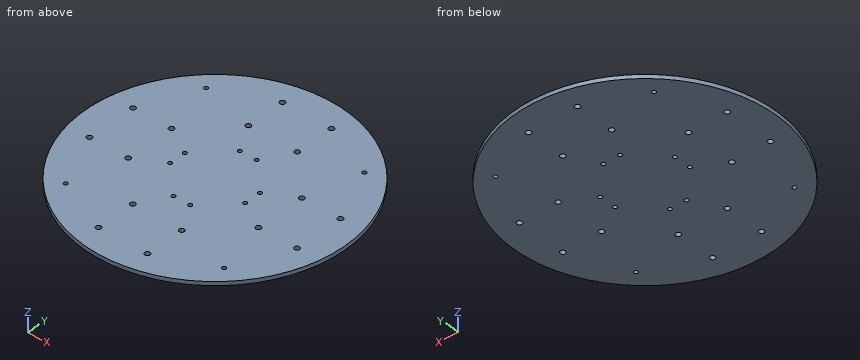
from build123d import *

# Parameters (mm, degrees)
CROQUIS1_R              = 100
CROQUIS1_R_2            = 2
SALIENTE_EXTRUIR1_DEPTH = 3
CORTAR_EXTRUIR2_START   = -3
CROQUIS2_R              = 2
CROQUIS2_R_2            = 1.5
CORTAR_EXTRUIR2_DEPTH   = 3
CROQUIS4_R              = 1.5
CORTAR_EXTRUIR3_DEPTH   = 3


with BuildPart() as part:
    # Croquis1 → Saliente-Extruir1 (new body)
    with BuildSketch(Plane.XY):
        Circle(CROQUIS1_R)
        with Locations((-50.610307618, 19)):
            Circle(CROQUIS1_R_2, mode=Mode.SUBTRACT)
        with Locations((-50.610307618, -19)):
            Circle(CROQUIS1_R_2, mode=Mode.SUBTRACT)
        with Locations((-80.610307618, 19)):
            Circle(CROQUIS1_R_2, mode=Mode.SUBTRACT)
        with Locations((-80.610307618, -19)):
            Circle(CROQUIS1_R_2, mode=Mode.SUBTRACT)
        with Locations((-19, -50.610307618)):
            Circle(CROQUIS1_R_2, mode=Mode.SUBTRACT)
        with Locations((19, -50.610307618)):
            Circle(CROQUIS1_R_2, mode=Mode.SUBTRACT)
        with Locations((-19, -80.610307618)):
            Circle(CROQUIS1_R_2, mode=Mode.SUBTRACT)
        with Locations((19, -80.610307618)):
            Circle(CROQUIS1_R_2, mode=Mode.SUBTRACT)
        with Locations((50.610307618, -19)):
            Circle(CROQUIS1_R_2, mode=Mode.SUBTRACT)
        with Locations((50.610307618, 19)):
            Circle(CROQUIS1_R_2, mode=Mode.SUBTRACT)
        with Locations((80.610307618, -19)):
            Circle(CROQUIS1_R_2, mode=Mode.SUBTRACT)
        with Locations((80.610307618, 19)):
            Circle(CROQUIS1_R_2, mode=Mode.SUBTRACT)
        with Locations((19, 50.610307618)):
            Circle(CROQUIS1_R_2, mode=Mode.SUBTRACT)
        with Locations((-19, 50.610307618)):
            Circle(CROQUIS1_R_2, mode=Mode.SUBTRACT)
        with Locations((19, 80.610307618)):
            Circle(CROQUIS1_R_2, mode=Mode.SUBTRACT)
        with Locations((-19, 80.610307618)):
            Circle(CROQUIS1_R_2, mode=Mode.SUBTRACT)
    extrude(amount=SALIENTE_EXTRUIR1_DEPTH)

    # Croquis2 → Cortar-Extruir2 (cut)
    with BuildSketch(Plane.XY.offset(3).offset(CORTAR_EXTRUIR2_START)):
        with Locations((19, 80.610307618)):
            Circle(CROQUIS2_R)
        with Locations((19, 50.610307618)):
            Circle(CROQUIS2_R)
        with Locations((-19, 50.610307618)):
            Circle(CROQUIS2_R)
        with Locations((-19, 80.610307618)):
            Circle(CROQUIS2_R)
        with Locations((-6.5, 29.110307618)):
            Circle(CROQUIS2_R_2)
        with Locations((6.5, 29.110307618)):
            Circle(CROQUIS2_R_2)
        with Locations((29.110307618, 6.5)):
            Circle(CROQUIS2_R_2)
        with Locations((29.110307618, -6.5)):
            Circle(CROQUIS2_R_2)
        with Locations((6.5, -29.110307618)):
            Circle(CROQUIS2_R_2)
        with Locations((-6.5, -29.110307618)):
            Circle(CROQUIS2_R_2)
        with Locations((-29.110307618, -6.5)):
            Circle(CROQUIS2_R_2)
        with Locations((-29.110307618, 6.5)):
            Circle(CROQUIS2_R_2)
    extrude(amount=CORTAR_EXTRUIR2_DEPTH, mode=Mode.SUBTRACT)

    # Croquis4 → Cortar-Extruir3 (cut)
    with BuildSketch(Plane.XY.offset(3)):
        with Locations((-61.518289963, 61.518289963)):
            Circle(CROQUIS4_R)
        with Locations((61.518289963, 61.518289963)):
            Circle(CROQUIS4_R)
        with Locations((61.518289963, -61.518289963)):
            Circle(CROQUIS4_R)
        with Locations((-61.518289963, -61.518289963)):
            Circle(CROQUIS4_R)
    extrude(amount=-CORTAR_EXTRUIR3_DEPTH, mode=Mode.SUBTRACT)


solid = part.part
Here's how the part is built. I have some questions about the finished solid (model axes, mm). Round coordinates to 2 decimals unless told otherwise and drop trailing zeros. Loops run counter-clockwise (first coordinate to the right, second up) from the corner with the lowest first, then second, coordinate; pieces in that order, holes last.
1. If we section it at A-A on z = 0.85: Count the separate pieces of the cut face and the enclosed holes in it, plus the area to 3 significant figures.
Answer list:
separate pieces: 1
enclosed holes: 28
area: 31,100 mm2
2. If I drill on line 1 along X through (y, z) = (82, 0.8); line 2 along Y through (x, z) = (6.5, 2.25); line 3 along Y through (x, z) = (-20, 2.5), over which ranges is the centre line in solid material (lowest first)?
Answer list:
line 1: x = -57.24 to -20.44, -17.56 to 17.56, 20.44 to 57.24
line 2: y = -99.79 to -30.61, -27.61 to 27.61, 30.61 to 99.79
line 3: y = -97.98 to -82.34, -78.88 to -52.34, -48.88 to 48.88, 52.34 to 78.88, 82.34 to 97.98
3. For P1, Ø2.5, axis at x = -19, y = -50.61, coming from the -Z side; P2, Ø1, axis at y = 16, z = 2, coming from the +X side, each with a flat end and sliding along its axis, tell me the tip position at first contact or that it passes through.
Answer list:
P1: passes through
P2: stops at x = 98.79
4. If we section it at C-C on y = 24: Write out the boundary of the cut face in (x, z).
Answer list:
outline: (-97.08, 0) - (97.08, 0) - (97.08, 3) - (-97.08, 3) - close
5. If we section it at B-B on x = -42: Write out the boundary of the cut face in (y, z), plus the area to 3 significant figures.
Answer list:
outline: (-90.75, 0) - (90.75, 0) - (90.75, 3) - (-90.75, 3) - close
area: 545 mm2
